Part model, mm, in its own coordinate system. A direction names the side the tool comes from. Coordinates: 2 decimals unless noted, no trailing zeros. Write each loop counter-clockwise with the first axis right and the second up, starting at its lowest first coordinate (ties: lowest second). Pieces come first, ordered by that corner, then holes. Notation, with made-up numbers: (-5, 0) -> (33, 0) arc R18 cw to (33, 29) -> close; hole circle Ø3 at (-28.75, -29). An arc over 180 degrees is marked (long way). Write item = value, one per line. Start each with the question number.
Q1. Pull direction X, two halves, no side cores. Call faces 6 (the flat face through (7, -50, 0)), 7 (the cylindrical face through (42.924, 1.201, -4.79)), 8 (the flat face through (-70, -1, 5)): released by +X, released by -X, zero draft, split by the parting line, or undercut.
Q2. Band-saw the part on D-D, the plane z = -15.5. List the corners of the cut face in (x, y), plus the area to 3 significant figures.
Q3. Tool access for faces 1 (the flat face through (-1, -57.5, 5)), 2 (the flat face through (4, -47.5, -10)), 3 (the flat face through (-60, -1, -10)), 4 (the cylindrical face through (76.803, 0.69, -10.14)), 5 (the flat face through (4, 47.5, -10)): list every direction of +Z, -Z, +X, -X, +Y, -Y with a clear straight run to the whole face (end or side of a thin tool).
Q4. Band-saw the part on C-C, the plane y = 42. List the corners of the cut face in (x, z), plus the area to 3 significant figures.
Q5. Band-saw the part on B-B, the plane z = 8.25. List the corners of the cut face in (x, y).
Q6. Band-saw the part on A-A, the plane x = -32.5. List the corners of the cut face in (y, z), plus the area to 3 significant figures.
Q7. Probe line 1 (X direction, y = -3.5, z = -14); line 2 (Z direction, x = 59, y = -51); line 3 (Y direction, x = 44.5, z = -16.25). List the from-to ranges inside material, lowest first.
Q8. Pin check, flat tips, straight feed: P1, Ø16, axis at y = 7, z = -11, coming from the -X side; P2, Ø6.5, axis at x = 39.11, y = 0, coming from the +Z side; P3, Ø12, axis at x = -46, z = -8.5, coming from the +Y side; P4, Ø5, axis at y = 26, z = -16, coming from the +X side. Stop position of each tip, or through.
from build123d import *

# Parameters (mm, degrees)
SKETCH_1_W          = 140
SKETCH_1_H          = 115
EXTRUDE_1_DEPTH     = 10
EXTRUDE_3_DEPTH     = 10
SKETCH_3_R          = 35
CUT_EXTRUDE_2_DEPTH = 10
SKETCH_4_R          = 35
EXTRUDE_4_DEPTH     = 10
SKETCH_5_R          = 4
CUT_EXTRUDE_3_DEPTH = 105.85349984
SKETCH_6_W          = 125.431788303
SKETCH_6_H          = 95
EXTRUDE_5_DEPTH     = 20
EXTRUDE_6_DEPTH     = 20
SKETCH_8_R          = 4
CUT_EXTRUDE_5_DEPTH = 107.274439207


with BuildPart() as part:
    # 草图1 → 凸台-拉伸1 (new body)
    with BuildSketch(Plane.XY):
        Rectangle(SKETCH_1_W, SKETCH_1_H)
    extrude(amount=EXTRUDE_1_DEPTH)

    # 草图2 → 凸台-拉伸3 (add)
    with BuildSketch(Plane.XY.offset(10)):
        with BuildLine():
            ThreePointArc((87.109163862, 0), (82.741171521, 29.995722562), (70, 57.5))
            Line((70, 57.5), (70, -57.5))
            ThreePointArc((70, -57.5), (82.741171521, -29.995722562), (87.109163862, 0))
        make_face()
    extrude(amount=-EXTRUDE_3_DEPTH)

    # 草图3 → 切除-拉伸2 (cut)
    with BuildSketch(Plane.XY.offset(10)):
        with Locations((37.109163862, 0)):
            Circle(SKETCH_3_R)
    extrude(amount=-CUT_EXTRUDE_2_DEPTH, mode=Mode.SUBTRACT)

    # 草图4 → 凸台-拉伸4 (add)
    with BuildSketch(Plane.XY.offset(10)):
        with Locations((37.109163862, 0)):
            Circle(SKETCH_4_R)
    extrude(amount=-EXTRUDE_4_DEPTH)

    # 草图5 → 切除-拉伸3 (cut, through all)
    with BuildSketch(Plane.XY.offset(10)):
        with Locations((39.109163862, 0)):
            Circle(SKETCH_5_R)
    extrude(amount=-CUT_EXTRUDE_3_DEPTH, mode=Mode.SUBTRACT)

    # 草图6 → 凸台-拉伸5 (add)
    with BuildSketch(Plane(origin=(0, 0, 0), x_dir=(-1, 0, 0), z_dir=(0, 0, -1))):
        with Locations((-2.715894151, 0)):
            Rectangle(SKETCH_6_W, SKETCH_6_H)
    extrude(amount=EXTRUDE_5_DEPTH)

    # 草图7 → 凸台-拉伸6 (add)
    with BuildSketch(Plane(origin=(0, 0, -20), x_dir=(-1, 0, 0), z_dir=(0, 0, -1))):
        with BuildLine():
            Line((-65.431788303, -47.5), (-65.431788303, 47.5))
            ThreePointArc((-65.431788303, 47.5), (-76.80558662, 0), (-65.431788303, -47.5))
        make_face()
    extrude(amount=-EXTRUDE_6_DEPTH)

    # 草图8 → 切除-拉伸5 (cut, through all)
    with BuildSketch(Plane.XY):
        with Locations((39.109163862, 0)):
            Circle(SKETCH_8_R)
    extrude(amount=-CUT_EXTRUDE_5_DEPTH, mode=Mode.SUBTRACT)


solid = part.part
Ans:
q1.face_6 = zero draft
q1.face_7 = undercut
q1.face_8 = released by -X
q2.outline = (-60, -47.5) -> (65.43, -47.5) arc R104.87 ccw to (65.43, 47.5) -> (-60, 47.5) -> close; hole circle Ø8 at (39.11, 0)
q2.area = 12,600 mm2
q3.face_1 = +Z, -Z, +X, -X, -Y
q3.face_2 = -Z, +X, -X, -Y
q3.face_3 = -Z, -X, +Y, -Y
q3.face_4 = -Z, +X
q3.face_5 = -Z, +X, -X, +Y
q4.outline = (-70, 0) -> (-60, 0) -> (-60, -20) -> (68.03, -20) -> (68.03, 0) -> (78.36, 0) -> (78.36, 10) -> (-70, 10) -> close
q4.area = 4,040 mm2
q5.outline = (-70, -57.5) -> (70, -57.5) arc R105.18 ccw to (70, 57.5) -> (-70, 57.5) -> close; hole circle Ø8 at (39.11, 0)
q6.outline = (-57.5, 0) -> (-47.5, 0) -> (-47.5, -20) -> (47.5, -20) -> (47.5, 0) -> (57.5, 0) -> (57.5, 10) -> (-57.5, 10) -> close
q6.area = 3,050 mm2
q7.line_1 = -60 to 37.17, 41.05 to 76.75
q7.line_2 = 0 to 10
q7.line_3 = -47.5 to 47.5
q8.P1 = -60
q8.P2 = through
q8.P3 = 47.5
q8.P4 = 74.14
